Design review of the part shown in the three views and the two pictorial views. Dimensions are in mm from the part's minimum x, y and z. Coordinates: 2 decimals unless noted, no trailing zeros. Loops run counter-clockwise (first coordinate to the right, second up) from the corner with the lowest first, then second, coordinate; pieces in that order, holes last. Notation, with made-up numbers: M 23.5,30.5 L 49.5,30.5 A30 ccw 49.5,64.5 Z; hole C -7,23 d10. An arc over 180 degrees is marked long. Put each result on its own line as item: value. Start each with the question number.
(1) Take a section at A-A, the plane z = 7. Give the boundary of the cut face in (x, y), then the cut area to 3 significant figures.
(2) For probe 1 along Z at (x, y) = (24.5, 2.15); probe 2 along X at (y, z) = (0.85, 105); probe 3 along Z at (x, y) = (16.5, 1.6), list the stretches that pass through material, from the lowest coordinate up. Write a range as [from, to].
(3) Take a section at D-D, the plane x = 4. Give the boundary of the cut face in (y, z), then the cut area to 3 significant figures.
(4) Take a section at C-C, the plane x = 34. Give the boundary of the cut face in (y, z).
(5) Take a section at B-B, the plane y = 1.35. Give the boundary of the cut face in (x, z).
(6) Clearance check with flat-ended pins moving along their axes: pin 1 (2 mm diameter, centred on x = 24.5, z = 105, fed in from +Y); pin 2 (1.5 mm diameter, centred on x = 15.5, y = 2, fed in from -Z); pin 3 (1 mm diameter, centred on x = 41, y = 2, fed in from +Z). State where each tip first meets the part, or that it passes through.
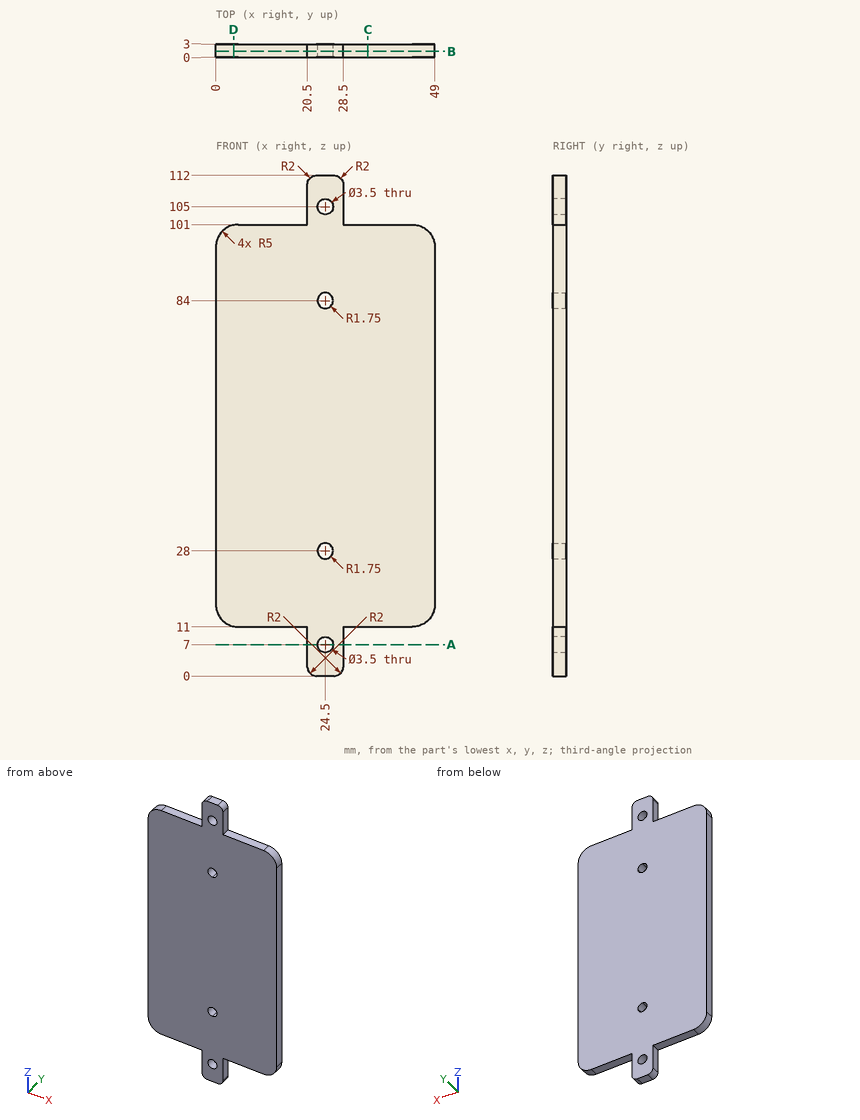
Computed values:
1. outline: M 20.5,0 L 22.75,0 L 22.75,3 L 20.5,3 Z; M 26.25,0 L 28.5,0 L 28.5,3 L 26.25,3 Z
1. area: 13.5 mm^2
2. probe 1: z = [0, 5.25], [8.75, 26.25], [29.75, 82.25], [85.75, 103.25], [106.75, 112]
2. probe 2: x = [20.5, 22.75], [26.25, 28.5]
2. probe 3: z = [11, 101]
3. outline: M 0,11.1 L 3,11.1 L 3,100.9 L 0,100.9 Z
3. area: 269 mm^2
4. outline: M 0,11 L 3,11 L 3,101 L 0,101 Z
5. outline: M 0,16 A5 ccw 5,11 L 20.5,11 L 20.5,2 A2 ccw 22.5,0 L 26.5,0 A2 ccw 28.5,2 L 28.5,11 L 44,11 A5 ccw 49,16 L 49,96 A5 ccw 44,101 L 28.5,101 L 28.5,110 A2 ccw 26.5,112 L 22.5,112 A2 ccw 20.5,110 L 20.5,101 L 5,101 A5 ccw 0,96 Z; hole C 24.5,7 d3.5; hole C 24.5,28 d3.5; hole C 24.5,84 d3.5; hole C 24.5,105 d3.5
6. pin 1: passes through
6. pin 2: stops at z = 11
6. pin 3: stops at z = 101
